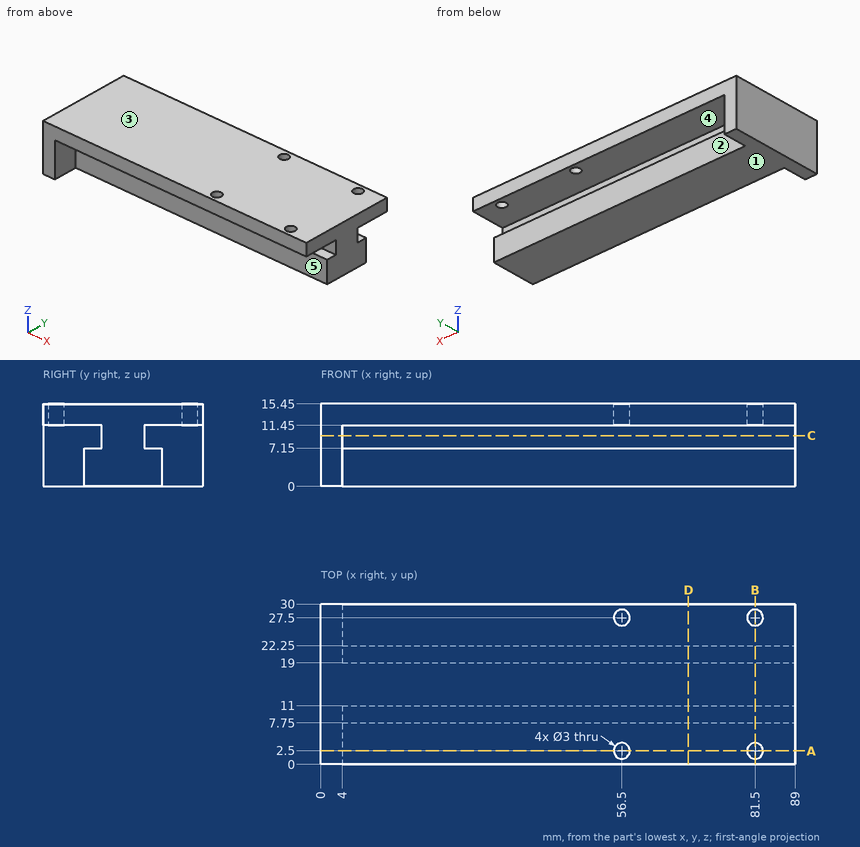
Check sheet for the drawn part. Datum: minimum x, y, z corner. Units: mm. A direction names the side the tool comes from. Round coordinates to 2 decimals unless told otherwise and drop trailing zeros. Order: outer loops, then holes, each group sorted by start corner. A loop starts at its lowest first (then second) coordinate and runs counter-clockwise, first axis right, second up.
(1) Cross-section at D-D, the plane x = 69. Enter the section's corners in (y, z), and give its area (3 significant figures).
(2) Scan lines: probe 1 along Y at (x, z) = (56.5, 12.8); probe 2 along X at (y, z) = (27.5, 13.65); probe 3 along Z at (x, y) = (13, 20.5). Record each from-to range of solid material in increasing order.
(3) Cross-section at C-C, the plane z = 9.5. Enter the section's corners in (x, y).
(4) Cross-section at A-A, the plane y = 2.5. Enter the section's corners in (x, z).
(5) Go/stop test with flat-tipped pins: P1, Ø2, axis at x = 41, z = 2.5, coming from the -Y side; P2, Ø1.3, axis at x = 67.5, z = 9, coming from the +Y side; P3, Ø2, axis at x = 66.5, z = 10, coming from the -Y side. Record where each tip stops, or that it passes through.
(6) Cross-section at B-B, the plane x = 81.5. Enter the section's corners in (y, z).
(7) Access from +Z, -Z, +X, -X, +Y, -Y to the whole of each face (thin tool, end or side, straight path). Record for the marked faces 1 and 2.
(8) Draft check along Z on the marked faces 3, 4 and 5. Enter one of: pulls with the +Z half, pulls with the -Z half, needs draft (parallel to the pull), parting line crosses it, or undercut.
Check sheet entries:
1. outline: (0, 11.45) - (11, 11.45) - (11, 7.15) - (7.75, 7.15) - (7.75, 0) - (22.25, 0) - (22.25, 7.15) - (19, 7.15) - (19, 11.45) - (30, 11.45) - (30, 15.45) - (0, 15.45) - close
1. area: 258 mm2
2. probe 1: y = 0 to 1, 4 to 26, 29 to 30
2. probe 2: x = 0 to 55, 58 to 80, 83 to 89
2. probe 3: z = 0 to 7.15, 11.45 to 15.45
3. outline: (0, 0) - (4, 0) - (4, 11) - (89, 11) - (89, 19) - (4, 19) - (4, 30) - (0, 30) - close
4. outline: (0, 0) - (4, 0) - (4, 11.45) - (55, 11.45) - (55, 15.45) - (0, 15.45) - close; (58, 11.45) - (80, 11.45) - (80, 15.45) - (58, 15.45) - close; (83, 11.45) - (89, 11.45) - (89, 15.45) - (83, 15.45) - close
5. P1: stops at y = 7.75
5. P2: stops at y = 19
5. P3: stops at y = 11
6. outline: (0, 11.45) - (1, 11.45) - (1, 15.45) - (0, 15.45) - close; (4, 11.45) - (11, 11.45) - (11, 7.15) - (7.75, 7.15) - (7.75, 0) - (22.25, 0) - (22.25, 7.15) - (19, 7.15) - (19, 11.45) - (26, 11.45) - (26, 15.45) - (4, 15.45) - close; (29, 11.45) - (30, 11.45) - (30, 15.45) - (29, 15.45) - close
7. face 1: -Z, +X, -X, +Y, -Y
7. face 2: -Z, +X, +Y
8. face 3: pulls with the +Z half
8. face 4: undercut
8. face 5: needs draft
